Verification items for the finished model (mm, model axes). A direction names the side the tool comes from. Coordinates: 2 decimals unless noted, no trailing zeros. Write each loop counter-clockwise with the first axis right and the second up, starting at its lowest first coordinate (ties: lowest second). Pieces come first, ordered by that corner, then holes. Notation, with made-up numbers: M -8,2.25 L 17,2.25 A17 ccw 17,31.25 Z; hole C -30.75,69 d8. An arc over 180 degrees is marked long. One line per item, written item: value.
```python
from build123d import *

# Parameters (mm, degrees)
SKETCH2_R           = 60
BOSS_EXTRUDE1_DEPTH = 360
SKETCH3_R           = 70
BOSS_EXTRUDE2_DEPTH = 10
BOSS_EXTRUDE4_DEPTH = 8


with BuildPart() as part:
    # Sketch2 → Boss-Extrude1 (new body)
    with BuildSketch(Plane.XY):
        Circle(SKETCH2_R)
    extrude(amount=BOSS_EXTRUDE1_DEPTH)

    # Sketch3 → Boss-Extrude2 (add)
    with BuildSketch(Plane(origin=(0, 0, 0), x_dir=(-1, 0, 0), z_dir=(0, 0, -1))):
        Circle(SKETCH3_R)
    extrude(amount=BOSS_EXTRUDE2_DEPTH)

    # Sketch4 → Boss-Extrude4 (add)
    with BuildSketch(Plane.XY.offset(360)):
        Polygon((-70, 120), (-120, 70), (-120, -70), (-70, -120), (70, -120), (120, -70), (120, 70), (70, 120), align=None)
    extrude(amount=BOSS_EXTRUDE4_DEPTH)


solid = part.part
```
Item 1: Cross-section at A-A, the plane y = 0. Enter the section's corners in (x, z).
The answers:
outline: M -120,360 L -60,360 L -60,0 L -70,0 L -70,-10 L 70,-10 L 70,0 L 60,0 L 60,360 L 120,360 L 120,368 L -120,368 Z
Item 2: Scan lines: line 1 (Z direction, x = 65, y = -15); line 2 (Z direction, x = 108, y = -81); line 3 (Y direction, x = -27, z = 7). Record each from-to range of solid material in increasing order.
The answers:
line 1: z = -10 to 0, 360 to 368
line 2: z = 360 to 368
line 3: y = -53.58 to 53.58
Item 3: Draft check along Z on faces 1 (the face through (-59.94, 2.64, 177.48)), 2 (the face through (-52, 31, 0)), 3 (the face through (-2, 2, 368)), 4 (the face through (-95, 95, 364)). Enter one of: released by +Z, released by -Z, zero draft, split by the parting line, or undercut.
The answers:
face 1: undercut
face 2: undercut
face 3: released by +Z
face 4: zero draft
Item 4: Access from +Z, -Z, +X, -X, +Y, -Y to the whole of each face (thin tool, end or side, straight path). Record for faces 5 (the face through (95, 95, 364)), 6 (the face through (55.55, -42.594, -4.93)).
The answers:
face 5: +Z, -Z, +X, +Y
face 6: -Z
Item 5: Cross-section at C-C, the plane z = 263. Enter the section's corners in (x, y), and give its area (3 significant figures).
The answers:
outline: C 0,0 d120
area: 11,300 mm²
Item 6: Go/stop test with flat-tipped pins: P1, Ø6, axis at x = 64, z = 245.5, coming from the -Y side; P2, Ø4, axis at x = 36, z = 228, coming from the +Y side; P3, Ø2, axis at x = -38.5, z = 171, coming from the -Y side; P4, Ø1.5, axis at y = -6.5, z = 307.5, coming from the -X side. Record where each tip stops, or that it passes through.
The answers:
P1: passes through
P2: stops at y = 49.44
P3: stops at y = -46.84
P4: stops at x = -59.72
Item 7: Cross-section at D-D, the plane y = 82. Enter the section's corners in (x, z).
The answers:
outline: M -108,360 L 108,360 L 108,368 L -108,368 Z
